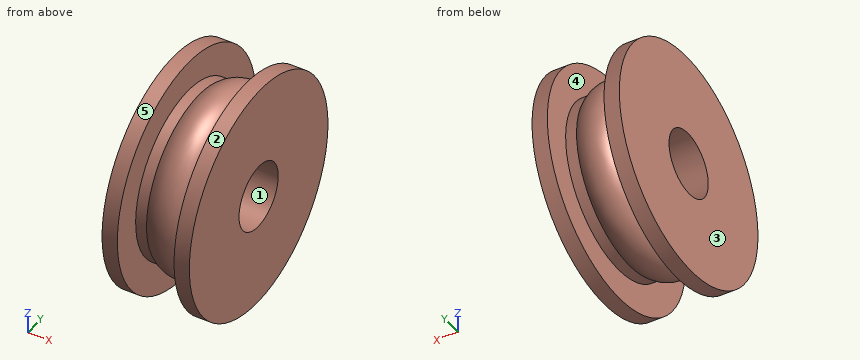
```python
from build123d import *

# Parameters (mm, degrees)
SKETCH2_R          = 1.5
CUT_EXTRUDE1_DEPTH = 9.495881355


with BuildPart() as part:
    # Sketch1 → Revolve1 (revolve)
    with BuildSketch(Plane.XY, mode=Mode.PRIVATE) as revolve1_sk:
        with BuildLine():
            Line((0, 0), (2, 0))
            Line((2, 0), (2, 5.3))
            Line((2, 5.3), (1.3, 5.3))
            Line((1.3, 5.3), (1.3, 3.9))
            Line((1.3, 3.9), (0.8, 3.9))
            ThreePointArc((0.8, 3.9), (0, 4.203250351), (-0.8, 3.9))
            Line((-0.8, 3.9), (-1.3, 3.9))
            Line((-1.3, 3.9), (-1.3, 5.3))
            Line((-1.3, 5.3), (-2, 5.3))
            Line((-2, 5.3), (-2, 0))
            Line((-2, 0), (0, 0))
        make_face()
    revolve(revolve1_sk.sketch.rotate(Axis((0, 0, 0), (1, 0, 0)), 90), axis=Axis((0, 0, 0), (1, 0, 0)))

    # Sketch2 → Cut-Extrude1 (cut, through all)
    with BuildSketch(Plane(origin=(2, 0, 0), x_dir=(0, 0, -1), z_dir=(1, 0, 0))):
        Circle(SKETCH2_R)
    extrude(amount=-CUT_EXTRUDE1_DEPTH, mode=Mode.SUBTRACT)


solid = part.part
```
The model under review builds one solid part; all positions refer to its coordinate system, in mm. Face numbers are marked on the shaded views. A direction names the side the tool comes from. Coordinates: 2 decimals unless noted, no trailing zeros. Order: outer loops, then holes, each group sorted by start corner. A loop starts at its lowest first (then second) coordinate and runs counter-clockwise, first axis right, second up. Notation, with made-up numbers: (53, 28) -> (90, 28) arc R23 ccw to (90, 39) -> close; hole circle Ø2 at (84.5, 0.25). An arc over 180 degrees is marked (long way). Answer in a Markdown table with one row per item. Add a question column.
Item 1: Clearance check with flat-ended pins moving along their axes: pin 1 (2 mm diameter, centred on x = 1, y = -3.5, fed in from -Z); pin 2 (2 mm diameter, centred on x = -1, y = -3, fed in from +Z). State where each tip first meets the part, or that it passes through.
Item 2: We need section D-D on x = -1.6. Write out the cut boundary in (y, z), plus the area to 3 significant figures.
Item 3: To check wall thickness, follow probe 1 along X at (y, z) = (4.75, -1.75); probe 2 along Y at (x, z) = (0.05, 0); probe 3 along Y at (x, z) = (-1.05, 0). State the ranges of each line that lie inside material, in increasing order.
Item 4: We need section C-C on x = -0.95. Write out the cut boundary in (y, z).
Item 5: We need section A-A on z = 0. Write out the cut boundary in (x, y), plus the area to 3 significant figures.
Item 6: Machinability: for the marked faces 4 and 5, which of the approach directions +Z, -Z, +X, -X, +Y, -Y give a long, thin tool a straight path to every point of the face, cutting with its end or side? Answer none if there is none.
Item 7: Mouldability with a two-part tool opening along Z and no side actions: class the marked faces 1, 2 and 3 as +Z half, -Z half, draft (parallel to the pull), parting line (faces both ways), or undercut.
Final values:
| question | item | result |
|---|---|---|
| 1 | pin 1 | stops at z = -4.65 |
| 1 | pin 2 | stops at z = 4.89 |
| 2 | outline | circle Ø10.6 at (0, 0); hole circle Ø3 at (0, 0) |
| 2 | area | 81.2 mm2 |
| 3 | probe 1 | x = -2 to -1.3, 1.3 to 2 |
| 3 | probe 2 | y = -4.2 to -1.5, 1.5 to 4.2 |
| 3 | probe 3 | y = -3.9 to -1.5, 1.5 to 3.9 |
| 4 | outline | circle Ø7.8 at (0, 0); hole circle Ø3 at (0, 0) |
| 5 | outline | (-2, -5.3) -> (-1.3, -5.3) -> (-1.3, -3.9) -> (-0.8, -3.9) arc R1.21 ccw to (0.8, -3.9) -> (1.3, -3.9) -> (1.3, -5.3) -> (2, -5.3) -> (2, -1.5) -> (-2, -1.5) -> close; (-2, 1.5) -> (2, 1.5) -> (2, 5.3) -> (1.3, 5.3) -> (1.3, 3.9) -> (0.8, 3.9) arc R1.21 ccw to (-0.8, 3.9) -> (-1.3, 3.9) -> (-1.3, 5.3) -> (-2, 5.3) -> close |
| 5 | area | 23.8 mm2 |
| 6 | face 4 | none |
| 6 | face 5 | +X, -X |
| 7 | face 1 | undercut |
| 7 | face 2 | parting line |
| 7 | face 3 | draft |
